from build123d import *

# Parameters (mm, degrees)
F0_W      = 80
F0_H      = 64
F0_W_2    = 42
F0_H_2    = 28
F1_DEPTH  = 3
F4_DEPTH  = 80
F5_T      = -2
F6_DEPTH  = 5
F7_R      = 1.5
F12_DEPTH = 2
F13_DEPTH = 2
F15_R     = 3.3298156999
F16_DEPTH = 25


# Not quite as in the source:
# - a feature names something its author has since deleted; it is built from what else it names


with BuildPart() as f1:
    # F0 (on Front) → F1 (new body)
    with BuildSketch(Plane.XZ):
        with Locations((-1, 1.9610269163)):
            Rectangle(F0_W, F0_H)
        with Locations((-7, 11.9610269163)):
            Rectangle(F0_W_2, F0_H_2, mode=Mode.SUBTRACT)
    extrude(amount=F1_DEPTH)

    # F3 (on offset) → F4 (join)
    with BuildSketch(Plane(origin=(-41, 0, 0), x_dir=(0, -1, 0), z_dir=(-1, 0, 0))):
        Polygon((0, -30.0389730837), (0, 33.9610269163), (-5, 33.9610269163), (-30.7466138076, 18.5625894163), (-5, -30.0389730837), align=None)
    extrude(amount=-F4_DEPTH)

    # F5
    f5_openings = [f1.faces().sort_by_distance(p)[0] for p in [
        (-1, 17.873307, -5.738192),
    ]]
    offset(amount=F5_T, openings=f5_openings, kind=Kind.INTERSECTION)

    # F0 (on Front) → F6 (cut)
    with BuildSketch(Plane.XZ):
        with Locations((-7, 11.9610269163)):
            Rectangle(F0_W_2, F0_H_2)
    extrude(amount=-F6_DEPTH, mode=Mode.SUBTRACT)

    # F7
    f7_edges = [f1.edges().sort_by_distance(p)[0] for p in [
        (39, -3, 1.961027),
        (39, 1, -30.038973),
        (-1, -3, -30.038973),
        (39, 1, 33.961027),
        (39, 17.873307, 26.261808),
        (-1, -3, 33.961027),
        (-1, 5, 33.961027),
        (-41, -3, 1.961027),
        (-41, 1, 33.961027),
        (-41, 17.873307, 26.261808),
        (-41, 1, -30.038973),
    ]]
    fillet(f7_edges, radius=F7_R)


with BuildPart() as f8_1:
    # F8: copy of F1
    add(f1.part)


with BuildPart() as f1_1:
    add(f1.part)

    # F11 (on offset) → F12 (join)
    with BuildSketch(Plane(origin=(0, 16.3302800697, -8.6509443873), x_dir=(-1, 0, 0), z_dir=(0, 0.8836647727, -0.468120251))):
        Polygon((-37, -15.9132964909), (-37, -21.9031590968), (39, -21.8151584268), (39, -15.9132964909), align=None)
    extrude(amount=-F12_DEPTH)

    # F11 (on offset) → F13 (join)
    with BuildSketch(Plane(origin=(0, 16.3302800697, -8.6509443873), x_dir=(-1, 0, 0), z_dir=(0, 0.8836647727, -0.468120251))):
        Polygon((39, 22.7937423885), (39, 28.7937423885), (-37, 28.7524405867), (-37, 22.7937423885), align=None)
    extrude(amount=-F13_DEPTH)

    # F15 (on offset) → F16 (cut)
    with BuildSketch(Plane(origin=(0, 16.2774082354, 27.2162772116), x_dir=(1, 0, 0), z_dir=(0, 0.51328125, 0.8582204603))):
        with Locations((0, 16.920266673)):
            Circle(F15_R)
    extrude(amount=-F16_DEPTH, mode=Mode.SUBTRACT)


solid = f1_1.part
Here's how the part is built. I have some questions about the finished solid (model axes, mm). A direction names the side the tool comes from. Give positions to 0.01 mm unless a question says otherwise; leave off trailing zeros. Order: outer loops, then holes, each group sorted by start corner. A loop starts at its lowest first (then second) coordinate and runs counter-clockwise, first axis right, second up. Notation, with made-up numbers: M 56,32.25 L 100,32.25 A27 cw 100,60.25 Z; hole C -16.75,6.5 d5. An arc over 180 degrees is marked long. Answer as a JSON object with one key per item and string values. Group by question number.
1) Please list where these lines run through material, in increasing order: L1, parallel to Z at x = 15.5, y = 1.5; L2, parallel to X at y = 0, z = 20; L3, parallel to Z at x = 3.5, y = -0.5. Write a range as [from, to].
2) Suppose I cut it at A-A, the plane y = 0. Write out the boundary of the cut face in (x, z).
3) Suppose I cut it at B-B, the plane x = 6.5. Count the separate pieces of the cut face and the enclosed holes in it, plus the area to 3 significant figures.
4) Suppose I cut it at D-D, the plane x = 33. Write out the boundary of the cut face in (y, z), plus the area to 3 significant figures.
5) On a 3-axis mill with a long thin cutter (end or side, diameter ignored), from which of +Z, -Z, +X, -X, +Y, -Y can I reach the whole of each face in a straight line? I mean faces 1 (the flat face through (16, 1, 12)), 2 (the flat face through (-7, 1, -4.039)), 3 (the flat face through (-20.7, 26.13, 11.95)), 4 (the flat face through (14, 0, 12)), 5 (the flat face through (-2, 2, 33.961)). Say none if no direction works.
6) Suppose I cut it at C-C, the plane z = 5.5. Write out the boundary of the cut face in (x, y).
7) I'm going to push flat-ended pins straight in: pin 1 Ø4 at (x, y) = (29, 15) entering from -Z; pin 2 Ø1.5 at (x, y) = (-30.5, 24.5) entering from +Z; pin 3 Ø6 at (x, y) = (-11.5, 21.5) entering from -Z; pin 4 Ø8 at (y, z) = (19.5, -10) entering from +X. Where does each tip first touch, or does it pass through?
8) We'd pull the mould along Y, two halves only. Please class faces 6 (the flat face through (-7, 0, -2.039)), 7 (the cylindrical face through (-40.572, 18.031, 25.642)), 8 (the flat face through (20.089, 26.652, 15.105)): pulls with the +Y half, pulls with the -Y half, needs draft (parallel to the pull), parting line crosses it, or undercut.
Results found:
{
 "1": {"L1": "[-30.04, -28.04], [-4.04, 27.96], [31.96, 33.96]", "L2": "[-41, -39], [-30, -28], [14, 16], [37, 39]", "L3": "[-30.04, -28.04], [-4.04, -2.04], [25.96, 27.96], [31.96, 33.96]"},
 "2": {"outline": "M -41,-28.54 A1.5 ccw -39.5,-30.04 L 37.5,-30.04 A1.5 ccw 39,-28.54 L 39,32.46 A1.5 ccw 37.5,33.96 L -39.5,33.96 A1.5 ccw -41,32.46 Z; M -30,-4.04 L 16,-4.04 L 16,27.96 L -30,27.96 Z; hole M -39,-28.04 L 37,-28.04 L 37,31.96 L -39,31.96 Z; hole M -28,-2.04 L 14,-2.04 L 14,25.96 L -28,25.96 Z"},
 "3": {"separate pieces": "4", "enclosed holes": "0", "area": "191 mm²"},
 "4": {"outline": "M -3,-28.54 A1.5 ccw -1.5,-30.04 L 5,-30.04 L 6.06,-28.04 L -1,-28.04 L -1,31.96 L 4.45,31.96 L 29.81,16.79 L 30.75,18.56 L 5.36,33.75 A1.5 ccw 4.59,33.96 L -1.5,33.96 A1.5 ccw -3,32.46 Z; M 4.31,-27.07 L 6.08,-28 L 8.88,-22.71 L 7.11,-21.78 Z; M 25.23,12.43 L 27,11.49 L 29.79,16.76 L 28.02,17.69 Z", "area": "235 mm²"},
 "5": {"face 1": "none", "face 2": "+Y", "face 3": "-Z", "face 4": "-Y", "face 5": "+Z, +X, -X, +Y, -Y"},
 "6": {"outline": "M -41,-1.5 A1.5 ccw -39.5,-3 L -28,-3 L -28,2 L -30,2 L -30,-1 L -39,-1 L -39,23.83 L -41,23.83 Z; M 14,-3 L 37.5,-3 A1.5 ccw 39,-1.5 L 39,23.83 L 37,23.83 L 37,-1 L 16,-1 L 16,2 L 14,2 Z"},
 "7": {"pin 1": "z = 24.45", "pin 2": "z = 22.75", "pin 3": "z = 19.97", "pin 4": "x = 39"},
 "8": {"face 6": "needs draft", "face 7": "pulls with the +Y half", "face 8": "undercut"}
}
